Geometry: final body of the model. Coordinates: model frame, mm. Face numbers are marked on the shaded views. Give positions to 0.01 mm unless a question says otherwise; leave off trailing zeros. Loops run counter-clockwise (first coordinate to the right, second up) from the corner with the lowest first, then second, coordinate; pieces in that order, holes last. Notation, with made-up numbers: (-11.75, 41) -> (20.25, 41) arc R16 ccw to (20.25, 56) -> close; hole circle Ø4 at (50.25, -26.5). An arc over 180 degrees is marked (long way). Answer in a Markdown table with one row per item. Add a question column.
from build123d import *

# Parameters (mm, degrees)
MAIN_BLOCK_SKETCH_W                                 = 70
MAIN_BLOCK_SKETCH_H                                 = 30
MAIN_BLOCK_DEPTH                                    = 20
NUT_TRAPS_DEPTH                                     = 2.4
TENSION_SCREW_HOLES_D                               = 3.4
CBORE_FOR_M5_HEX_SOCKET_HEAD_CAP_SCREW1_D           = 5.5
CBORE_FOR_M5_HEX_SOCKET_HEAD_CAP_SCREW1_CBORE_D     = 10
CBORE_FOR_M5_HEX_SOCKET_HEAD_CAP_SCREW1_CBORE_DEPTH = 5.4
PRINT_HELPER_FILLETS_R                              = 2
COSMETIC_CHAMFER_SIZE                               = 2


with BuildPart() as part:
    # Main Block Sketch → Main Block (new body)
    with BuildSketch(Plane(origin=(0, 0, 0), x_dir=(1, 0, 0), z_dir=(0, 1, 0))):
        with Locations((0, -15)):
            Rectangle(MAIN_BLOCK_SKETCH_W, MAIN_BLOCK_SKETCH_H)
    extrude(amount=MAIN_BLOCK_DEPTH)

    # Nut TrapsSketch → Nut Traps (cut)
    with BuildSketch(Plane(origin=(0, 20, 0), x_dir=(1, 0, 0), z_dir=(0, 1, 0))):
        Polygon((-15.825684219, -19.6), (-19.174315781, -19.6), (-20.848631561, -22.5), (-19.174315781, -25.4), (-15.825684219, -25.4), (-14.151368439, -22.5), align=None)
        Polygon((19.174315781, -19.6), (15.825684219, -19.6), (14.151368439, -22.5), (15.825684219, -25.4), (19.174315781, -25.4), (20.848631561, -22.5), align=None)
    extrude(amount=-NUT_TRAPS_DEPTH, mode=Mode.SUBTRACT)

    # Tension Screw Holes (through all)
    with Locations(Plane(origin=(0, 20, 0), x_dir=(1, 0, 0), z_dir=(0, 1, 0))):
        with Locations((-17.5, -22.5), (17.5, -22.5)):
            Hole(TENSION_SCREW_HOLES_D / 2)

    # CBORE for M5 Hex Socket Head Cap Screw1 (through all)
    with Locations(Plane.XY.offset(30)):
        with Locations((-27.5, 10), (27.5, 10)):
            CounterBoreHole(CBORE_FOR_M5_HEX_SOCKET_HEAD_CAP_SCREW1_D / 2, CBORE_FOR_M5_HEX_SOCKET_HEAD_CAP_SCREW1_CBORE_D / 2, CBORE_FOR_M5_HEX_SOCKET_HEAD_CAP_SCREW1_CBORE_DEPTH)

    # Print Helper Fillets
    print_helper_fillets_edges = [part.edges().sort_by_distance(p)[0] for p in [
        (35, 10, 30),
        (35, 10, 0),
        (-35, 10, 0),
        (-35, 10, 30),
    ]]
    fillet(print_helper_fillets_edges, radius=PRINT_HELPER_FILLETS_R)

    # Cosmetic Chamfer
    cosmetic_chamfer_edges = [part.edges().sort_by_distance(p)[0] for p in [
        (35, 20, 15),
        (0, 20, 30),
        (0, 20, 0),
        (-35, 20, 15),
        (-34.414213562, 20, 29.414213562),
        (-34.414213562, 20, 0.585786438),
        (34.414213562, 20, 0.585786438),
        (34.414213562, 20, 29.414213562),
    ]]
    chamfer(cosmetic_chamfer_edges, length=COSMETIC_CHAMFER_SIZE)


solid = part.part
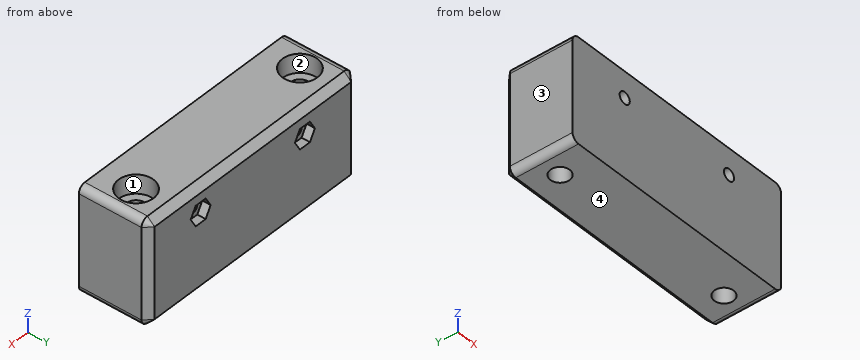
(1) Material intervals for line 1 along X through (y, z) = (14, 22.5); line 2 along Y through (x, z) = (27.5, 8.25); line 3 along X through (y, z) = (11.25, 19.5), sorted ascending. Write a range as from..to.
(2) Cut plane C-C on z = 8.25. Return the cut outline in (x, y), then the cut area to 3 significant figures.
(3) Cut plane B-B on x = -17.5. Return the cut outline in (y, z).
(4) Pin query (flat end, axial travel): pin 1 Ø1.9 at (x, y) = (-17, 19) entering from -Z; pin 2 Ø0.7 at (x, y) = (17.5, 18.5) entering from +Z; pin 3 Ø4 at (x, z) = (-17.5, 22.5) entering from +Y. Return the tip coordinate at first contact, or that it passes through.
(5) Cut plane A-A on y = 10. Return the cut outline in (x, z).
(6) Cut plane D-D on x = -27.5. Return the cut outline in (y, z).
(7) Draft query along X for the marked faces 1, 2, 3 and 4. Return one class per face: +X half, -X half, draft (parallel to the pull), parting line (faces both ways), or undercut.
Answer list:
| question | item | result |
|---|---|---|
| 1 | line 1 | x = -35..-19.2, -15.8..15.8, 19.2..35 |
| 1 | line 2 | y = 0..7.25, 12.75..20 |
| 1 | line 3 | x = -35..-29.95, -25.05..25.05, 29.95..35 |
| 2 | outline | (-35, 0) -> (35, 0) -> (35, 18) -> (33, 20) -> (-33, 20) -> (-35, 18) -> close; hole circle Ø5.5 at (-27.5, 10); hole circle Ø5.5 at (27.5, 10) |
| 2 | area | 1,350 mm² |
| 3 | outline | (0, 0) -> (18, 0) -> (20, 2) -> (20, 19.6) -> (17.6, 19.6) -> (17.6, 20.8) -> (0, 20.8) -> close; (0, 24.2) -> (17.6, 24.2) -> (17.6, 25.4) -> (20, 25.4) -> (20, 28) -> (18, 30) -> (0, 30) -> close |
| 4 | pin 1 | stops at z = 0.05 |
| 4 | pin 2 | stops at z = 29.85 |
| 4 | pin 3 | stops at y = 17.6 |
| 5 | outline | (-35, 2) arc R2 ccw to (-33, 0) -> (-30.25, 0) -> (-30.25, 24.6) -> (-32.5, 24.6) -> (-32.5, 30) -> (-33, 30) arc R2 ccw to (-35, 28) -> close; (-24.75, 0) -> (24.75, 0) -> (24.75, 24.6) -> (22.5, 24.6) -> (22.5, 30) -> (-22.5, 30) -> (-22.5, 24.6) -> (-24.75, 24.6) -> close; (30.25, 0) -> (33, 0) arc R2 ccw to (35, 2) -> (35, 28) arc R2 ccw to (33, 30) -> (32.5, 30) -> (32.5, 24.6) -> (30.25, 24.6) -> close; hole circle Ø3.4 at (-17.5, 22.5); hole circle Ø3.4 at (17.5, 22.5) |
| 6 | outline | (0, 0) -> (7.25, 0) -> (7.25, 24.6) -> (5, 24.6) -> (5, 30) -> (0, 30) -> close; (12.75, 0) -> (18, 0) -> (20, 2) -> (20, 28) -> (18, 30) -> (15, 30) -> (15, 24.6) -> (12.75, 24.6) -> close |
| 7 | face 1 | undercut |
| 7 | face 2 | undercut |
| 7 | face 3 | -X half |
| 7 | face 4 | draft |
